Design review of the part shown in the three views and the two pictorial views. Dimensions are in mm from the part's minimum x, y and z. A direction names the side the tool comes from. Round coordinates to 2 decimals unless told otherwise and drop trailing zeros. Write each loop counter-clockwise with the first axis right and the second up, starting at its lowest first coordinate (ties: lowest second). Pieces come first, ordered by that corner, then holes. Notation, with made-up numbers: (32.5, 2.5) -> (37.5, 2.5) arc R27 ccw to (37.5, 41.5) -> close; hole circle Ø4 at (89.25, 88.5). An arc over 180 degrees is marked (long way). Answer as a JSON object with one key per item and string values. Group by question number.
1) To check wall thickness, follow probe 1 along X at (y, z) = (1.6, 18); probe 2 along X at (y, z) = (8.5, 18.5); probe 3 along X at (y, z) = (60, 6). State the ranges of each line that lie inside material, in increasing order. Write a range as [from, to].
2) We need section C-C, the plane y = 50. Write out the cut boundary in (x, z), then the cut area to 3 significant figures.
3) Mouldability with a two-part tool opening along Y and no side actions: class the marked faces 1, 2 and 3 as pulls with the +Y half, pulls with the -Y half, needs draft (parallel to the pull), parting line crosses it, or undercut.
4) Insertion check: pin 1 Ø7.5 at (y, z) = (32, 20) entering from +X; pin 2 Ø5 at (x, y) = (17.5, 53.5) entering from -Z; pin 3 Ø6.5 at (x, y) = (19.5, 43) entering from +Z. Each pin has a flat end and moves straight along its axis. Give the tip position at first contact, or say it passes through.
5) Machinability: for the marked faces 4, 5 and 6, which of the approach directions +Z, -Z, +X, -X, +Y, -Y give a long, thin tool a straight path to every point of the face, cutting with its end or side? Answer none if there is none.
6) We need section A-A, the plane z = 18. Write out the cut boundary in (x, y), then the cut area to 3 significant figures.
7) We need section B-B, the plane x = 28. Write out the cut boundary in (y, z).
8) We need section D-D, the plane x = 17.5. Write out the cut boundary in (y, z).
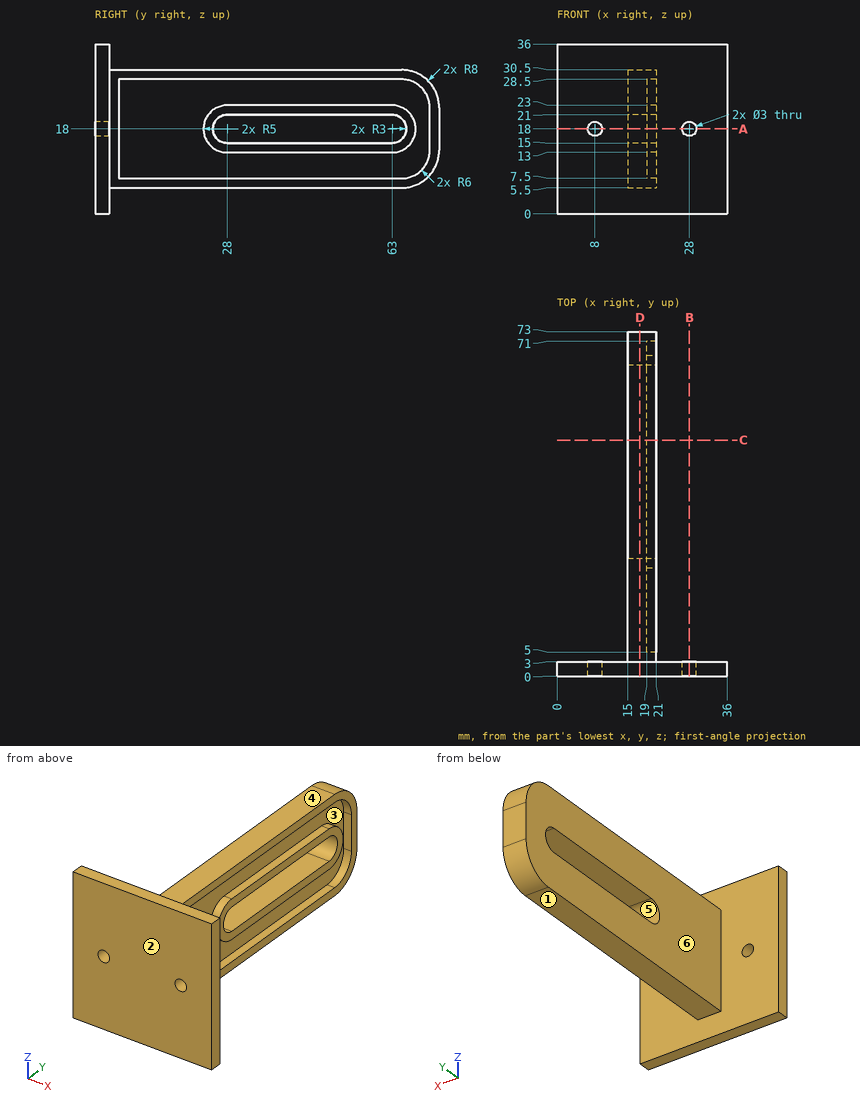
Here are the results:
{
 "1": {"probe 1": "x = [0, 6.5], [9.5, 26.5], [29.5, 36]", "probe 2": "x = [15, 19]", "probe 3": "x = [15, 21]"},
 "2": {"outline": "(15, 5.5) -> (21, 5.5) -> (21, 7.5) -> (19, 7.5) -> (19, 13) -> (21, 13) -> (21, 15) -> (15, 15) -> close; (15, 21) -> (21, 21) -> (21, 23) -> (19, 23) -> (19, 28.5) -> (21, 28.5) -> (21, 30.5) -> (15, 30.5) -> close", "area": "92.0 mm^2"},
 "3": {"face 1": "needs draft", "face 2": "pulls with the -Y half", "face 3": "undercut"},
 "4": {"pin 1": "stops at x = 21", "pin 2": "stops at z = 5.5", "pin 3": "stops at z = 30.5"},
 "5": {"face 4": "+Z, +X, -X, +Y", "face 5": "+X, -X", "face 6": "+Z, -Z, -X, +Y"},
 "6": {"outline": "(0, 0) -> (6.5, 0) -> (6.5, 3) -> (0, 3) -> close; (9.5, 0) -> (26.5, 0) -> (26.5, 3) -> (21, 3) -> (21, 5) -> (19, 5) -> (19, 23) -> (21, 23) -> (21, 25) -> (15, 25) -> (15, 3) -> (9.5, 3) -> close; (15, 66) -> (21, 66) -> (21, 68) -> (19, 68) -> (19, 71) -> (21, 71) -> (21, 73) -> (15, 73) -> close; (29.5, 0) -> (36, 0) -> (36, 3) -> (29.5, 3) -> close", "area": "222 mm^2"},
 "7": {"outline": "(0, 0) -> (3, 0) -> (3, 16.5) -> (0, 16.5) -> close; (0, 19.5) -> (3, 19.5) -> (3, 36) -> (0, 36) -> close"},
 "8": {"outline": "(0, 0) -> (3, 0) -> (3, 5.5) -> (65, 5.5) arc R8 ccw to (73, 13.5) -> (73, 22.5) arc R8 ccw to (65, 30.5) -> (3, 30.5) -> (3, 36) -> (0, 36) -> close; hole (28, 15) -> (63, 15) arc R3 ccw to (63, 21) -> (28, 21) arc R3 ccw to start"}
}
